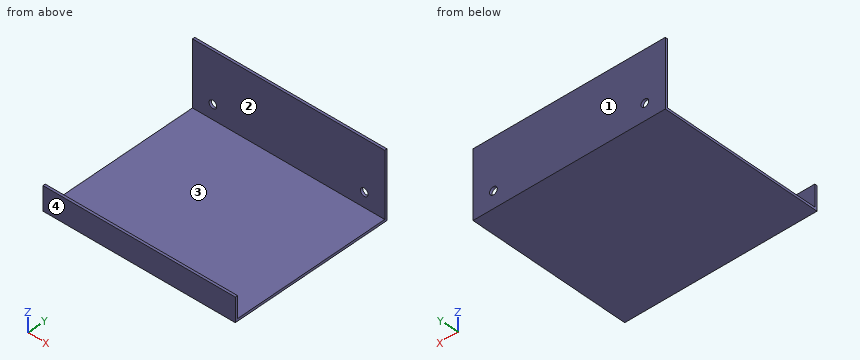
from build123d import *

# Parameters (mm, degrees)
SKETCH_W        = 80
SKETCH_H        = 68
PAD_DEPTH       = 28
SKETCH001_W     = 66
SKETCH001_H     = 27
POCKET_DEPTH    = 80
SKETCH002_W     = 1
SKETCH002_H     = 18
POCKET001_DEPTH = 80
SKETCH003_R     = 1.6
POCKET002_DEPTH = 5


with BuildPart() as part:
    # Sketch → Pad (new body)
    with BuildSketch(Plane.XY):
        with Locations((40, 34)):
            Rectangle(SKETCH_W, SKETCH_H)
    extrude(amount=PAD_DEPTH)

    # Sketch001 (on Face4 of Pad) → Pocket (cut)
    with BuildSketch(Plane(origin=(0, 0, 0), x_dir=(0, -1, 0), z_dir=(-1, 0, 0))):
        with Locations((-34, 14.5)):
            Rectangle(SKETCH001_W, SKETCH001_H)
    extrude(amount=-POCKET_DEPTH, mode=Mode.SUBTRACT)

    # Sketch002 (on Face2 of Pocket) → Pocket001 (cut)
    with BuildSketch(Plane(origin=(0, 0, 0), x_dir=(0, -1, 0), z_dir=(-1, 0, 0))):
        with Locations((-0.5, 19)):
            Rectangle(SKETCH002_W, SKETCH002_H)
    extrude(amount=-POCKET001_DEPTH, mode=Mode.SUBTRACT)

    # Sketch003 (on Face6 of Pocket001) → Pocket002 (cut)
    with BuildSketch(Plane(origin=(0, 68, 0), x_dir=(-1, 0, 0), z_dir=(0, 1, 0))):
        with Locations((-71.5, 7)):
            Circle(SKETCH003_R)
        with Locations((-8.5, 7)):
            Circle(SKETCH003_R)
    extrude(amount=-POCKET002_DEPTH, mode=Mode.SUBTRACT)


solid = part.part
The listing builds one solid part. Answer for the finished solid, in the listing's coordinates (mm). Face numbers are marked on the shaded views. Round coordinates to 2 decimals unless told otherwise and drop trailing zeros. Order: outer loops, then holes, each group sorted by start corner. A loop starts at its lowest first (then second) coordinate and runs counter-clockwise, first axis right, second up. Notation, with made-up numbers: (37.5, -33.75) -> (87.5, -33.75) arc R18 cw to (87.5, -8.75) -> close; hole circle Ø8 at (28.5, 48.5). An arc over 180 degrees is marked (long way). Put each result on its own line as item: value.
Q1. Consider line 1 along Y through (x, z) = (44, 4); line 2 along Z through (x, y) = (8.5, 67.45); line 3 along Y through (x, z) = (29, 14). Determine where each line is inside the solid, lowest interval first.
Results list:
line 1: 0 to 1, 67 to 68
line 2: 0 to 5.4, 8.6 to 28
line 3: 67 to 68
Q2. Section C-C, the plane y = 55.5 is taken. Write down the section's boundary in (x, z).
Results list:
outline: (0, 0) -> (80, 0) -> (80, 1) -> (0, 1) -> close
Q3. Each of these flat-tipped pins is pushed along its axis until it touches: P1, Ø3, axis at x = 54, y = 47.5, coming from the +Z side; P2, Ø0.5, axis at x = 31, y = 0.5, coming from the +Z side; P3, Ø13.5, axis at x = 53, z = 20, coming from the -Y side. Where does it stop, or does it pass through?
Results list:
P1: z = 1
P2: z = 10
P3: y = 67
Q4. Determine the mould class of the marked faces 1, 2, 3 and 4 for opening direction Y: pulls with the +Y half, pulls with the -Y half, needs draft (parallel to the pull), parting line crosses it, or undercut.
Results list:
face 1: pulls with the +Y half
face 2: undercut
face 3: undercut
face 4: pulls with the -Y half
Q5. Section A-A, the plane z = 7 is taken. Write down the section's boundary in (x, y).
Results list:
outline: (0, 0) -> (80, 0) -> (80, 1) -> (0, 1) -> close; (0, 67) -> (6.9, 67) -> (6.9, 68) -> (0, 68) -> close; (10.1, 67) -> (69.9, 67) -> (69.9, 68) -> (10.1, 68) -> close; (73.1, 67) -> (80, 67) -> (80, 68) -> (73.1, 68) -> close
Q6. Section D-D, the plane z = 11.5 is taken. Write down the section's boundary in (x, y).
Results list:
outline: (0, 67) -> (80, 67) -> (80, 68) -> (0, 68) -> close
Q7. Section B-B, the plane x = 71.5 is taken. Write down the section's boundary in (y, z).
Results list:
outline: (0, 0) -> (68, 0) -> (68, 5.4) -> (67, 5.4) -> (67, 1) -> (1, 1) -> (1, 10) -> (0, 10) -> close; (67, 8.6) -> (68, 8.6) -> (68, 28) -> (67, 28) -> close
